Geometry check sheet. Reference: drawing and pictorial views, mm from the part's lowest x, y, z. A direction names the side the tool comes from. Round coordinates to 2 decimals unless told otherwise and drop trailing zeros. Loops run counter-clockwise (first coordinate to the right, second up) from the corner with the lowest first, then second, coordinate; pieces in that order, holes last. Notation, with made-up numbers: (-34.75, 14.25) - (10.25, 14.25) arc R19 cw to (10.25, 18.25) - close; hole circle Ø6 at (83.5, 6). An arc over 180 degrees is marked (long way). Put each result on its own line as item: value. Start each with the question number.
Item 1: Material ranges on line 1 along Z through (x, y) = (5, 0.6); line 2 along Y through (x, z) = (4.5, 11), recorded low to high.
Item 2: Tool access check on the marked faces 1, 2 and 3. Record the directions out of +Z, -Z, +X, -X, +Y, -Y that give a thin tool (end or side, any length) a straight path to the whole face; none if there is none.
Item 3: Draft check along X on the marked faces 4, 5 and 6. Enter one of: pulls with the +X half, pulls with the -X half, needs draft (parallel to the pull), parting line crosses it, or undercut.
Item 4: Section check A-A, the plane x = 5. Record the cut outline in (y, z).
Item 5: Section check C-C, the plane y = 8.5. Record the cut outline in (x, z).
Item 6: Gauge pin test, flat ends, axial feed: pin 1 Ø5 at (x, z) = (5, 11.5) entering from +Y; pin 2 Ø3.5 at (x, y) = (5.5, 8) entering from +Z. Record the tip position at first contact, or that the pin passes through.
Item 7: Section check D-D, the plane y = 5.25. Record the cut outline in (x, z).
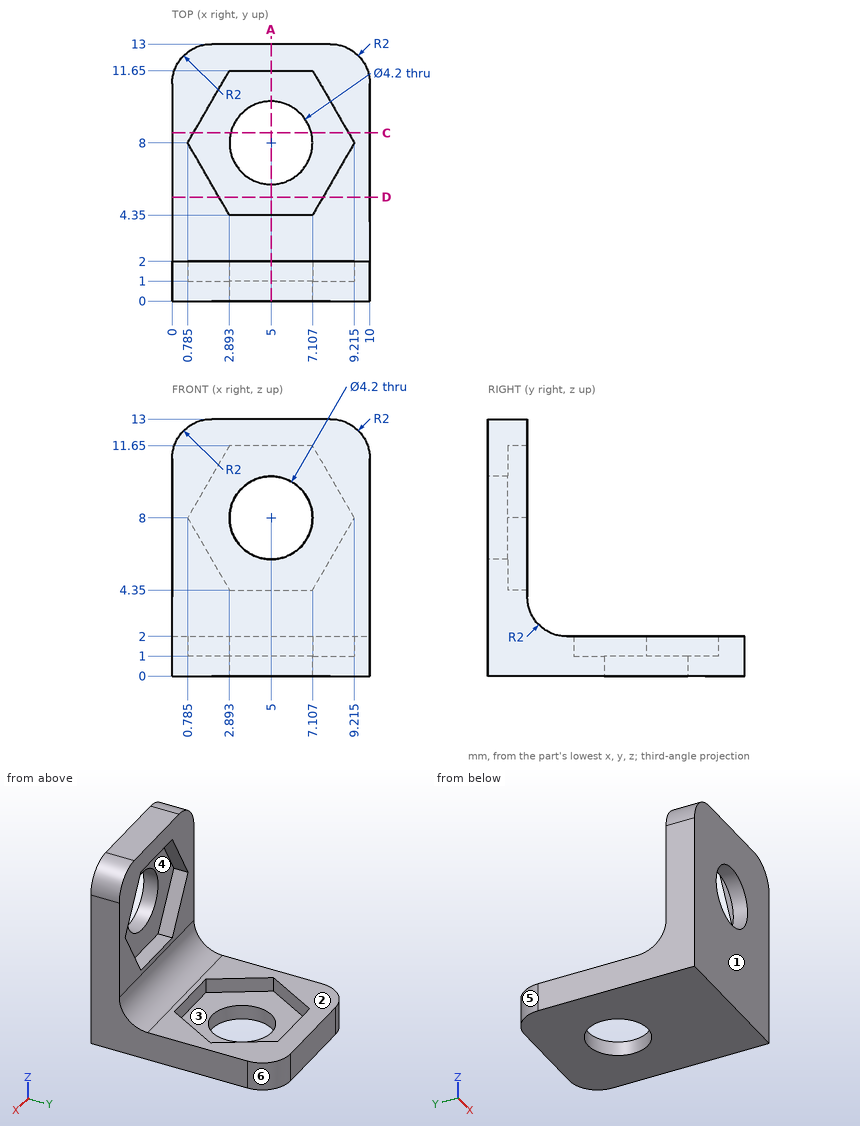
Check result:
1. line 1: 0 to 5.9, 10.1 to 13
1. line 2: 0 to 1
2. face 1: +Z, -Z, +X, -X, -Y
2. face 2: +Z, +X, -X, +Y
2. face 3: +Z
3. face 4: undercut
3. face 5: pulls with the -X half
3. face 6: pulls with the +X half
4. outline: (0, 0) - (5.9, 0) - (5.9, 1) - (4.35, 1) - (4.35, 2) - (4, 2) arc R2 cw to (2, 4) - (2, 4.35) - (1, 4.35) - (1, 5.9) - (0, 5.9) - close; (0, 10.1) - (1, 10.1) - (1, 11.65) - (2, 11.65) - (2, 13) - (0, 13) - close; (10.1, 0) - (13, 0) - (13, 2) - (11.65, 2) - (11.65, 1) - (10.1, 1) - close
5. outline: (0, 0) - (2.96, 0) - (2.96, 1) - (1.07, 1) - (1.07, 2) - (0, 2) - close; (7.04, 0) - (10, 0) - (10, 2) - (8.93, 2) - (8.93, 1) - (7.04, 1) - close
6. pin 1: y = 2
6. pin 2: z = 1
7. outline: (0, 0) - (10, 0) - (10, 2) - (7.63, 2) - (7.63, 1) - (2.37, 1) - (2.37, 2) - (0, 2) - close
